Study the drawing (mm; zero at the part's minimum x, y, z) and answer. A direction names the side the tool comes from. Coordinates: 2 decimals unless noted, no trailing zeros. Order: outer loops, then holes, each group sorted by start corner. A loop starts at its lowest first (then second) coordinate and runs counter-clockwise, first axis right, second up. Notation, with made-up numbers: (34, 68) -> (90, 68) arc R29 ccw to (90, 101) -> close; hole circle Ø5 at (8.25, 6). An arc over 180 degrees is marked (long way). Answer in a Markdown table with one row per item. Add a question column.
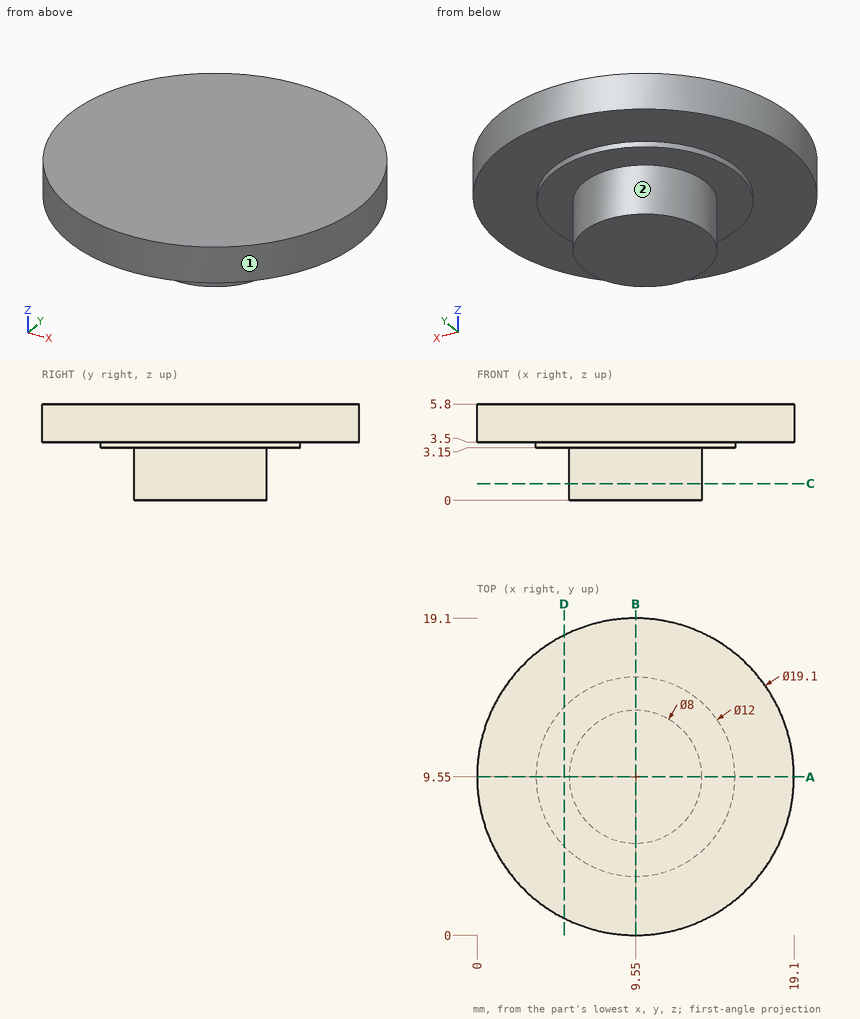
Q1. A cutting plane is placed at D-D (x = 5.25). Determine the outline of the cut face in (y, z), then the cut area to 3 significant figures.
Q2. Straight lines are drawn through the part: line 1 (Z direction, x = 16, y = 2.75); line 2 (Y direction, x = 7, z = 4.6); line 3 (X direction, y = 3.25, z = 4.35). For each, find the intervals that lie inside material, in ascending order.
Q3. A cutting plane is placed at C-C (z = 1). Determine the outline of the cut face in (x, y).
Q4. A cutting plane is placed at A-A (y = 9.55). Determine the outline of the cut face in (x, z), then the cut area to 3 significant figures.
Q5. Given pin 1 (3 mm diameter, centred on y = 17, z = 4.5, fed in from +X); pin 2 (5 mm diameter, centred on x = 3, y = 5.5, fed in from -Z), each flat-ended and moving along its own axis, determine where each tip first touches the part or whether it passes through.
Q6. For the marked faces 1 and 2, determine the directions among +Z, -Z, +X, -X, +Y, -Y from which every point of the face is accessible in a straight line to the end or side of a thin tool.
Returned:
| question | item | result |
|---|---|---|
| 1 | outline | (1.02, 3.5) -> (5.37, 3.5) -> (5.37, 3.15) -> (13.73, 3.15) -> (13.73, 3.5) -> (18.08, 3.5) -> (18.08, 5.8) -> (1.02, 5.8) -> close |
| 1 | area | 42.2 mm² |
| 2 | line 1 | z = 3.5 to 5.8 |
| 2 | line 2 | y = 0.35 to 18.75 |
| 2 | line 3 | x = 2.37 to 16.73 |
| 3 | outline | circle Ø8 at (9.55, 9.55) |
| 4 | outline | (0, 3.5) -> (3.55, 3.5) -> (3.55, 3.15) -> (5.55, 3.15) -> (5.55, 0) -> (13.55, 0) -> (13.55, 3.15) -> (15.55, 3.15) -> (15.55, 3.5) -> (19.1, 3.5) -> (19.1, 5.8) -> (0, 5.8) -> close |
| 4 | area | 73.3 mm² |
| 5 | pin 1 | stops at x = 17.02 |
| 5 | pin 2 | stops at z = 3.15 |
| 6 | face 1 | +Z, -Z |
| 6 | face 2 | -Z |
